Geometry: final body of the model. Coordinates: model frame, mm. Give positions to 0.01 mm unless a question says otherwise; leave off trailing zeros. Write each loop counter-clockwise with the first axis right and the second up, starting at its lowest first coordinate (ties: lowest second). Pieces come first, ordered by that corner, then holes. Notation, with made-up numbers: (-28.75, -36) - (-1.75, -36) arc R13 cw to (-1.75, -14) - close; hole circle Ø1 at (28, 46). An arc over 180 degrees is marked (long way). Return JSON: item names as keys, results as strings.
from build123d import *

# Parameters (mm, degrees)
BOSS_EXTRUDE1_DEPTH            = 9.525
CUT_EXTRUDE1_REACH             = 11.525
SKETCH2_R                      = 2.54
SKETCH2_W                      = 6.35
SKETCH2_H                      = 30
CUT_EXTRUDE2_REACH             = 230.6
SKETCH3_R                      = 2.2479
F_7_0_201_DIAMETER_HOLE1_D     = 5.1054
F_7_0_201_DIAMETER_HOLE1_DEPTH = 3.175
F_7_0_201_DIAMETER_HOLE1_TIP   = 1.533816902
SKETCH7_R                      = 6.35
CUT_EXTRUDE3_DEPTH             = 10.525


with BuildPart() as part:
    # Sketch1 → Boss-Extrude1 (new body)
    with BuildSketch(Plane(origin=(0, 0, 0), x_dir=(1, 0, 0), z_dir=(0, 1, 0))):
        with BuildLine():
            Line((6.35, 0), (101.6, 0))
            ThreePointArc((101.6, 0), (155.481536726, -22.318463274), (177.8, -76.2))
            Line((177.8, -76.2), (177.8, -228.6))
            ThreePointArc((177.8, -228.6), (203.2, -254), (228.6, -228.6))
            Line((228.6, -228.6), (228.6, 241.3))
            ThreePointArc((228.6, 241.3), (224.880256121, 250.280256121), (215.9, 254))
            Line((215.9, 254), (6.35, 254))
            ThreePointArc((6.35, 254), (1.859871939, 252.140128061), (0, 247.65))
            Line((0, 247.65), (0, 6.35))
            ThreePointArc((0, 6.35), (1.859871939, 1.859871939), (6.35, 0))
        make_face()
    extrude(amount=BOSS_EXTRUDE1_DEPTH)

    # Sketch2 → Cut-Extrude1 (cut, up to next)
    with BuildSketch(Plane(origin=(0, 9.525, 0), x_dir=(1, 0, 0), z_dir=(0, 1, 0)), mode=Mode.PRIVATE) as cut_extrude1_sk1:
        with Locations((28.34999918, 213.6)):
            Circle(SKETCH2_R)
    cut_extrude1_tool1 = extrude(cut_extrude1_sk1.sketch, amount=-CUT_EXTRUDE1_REACH, mode=Mode.PRIVATE) & part.part
    add(cut_extrude1_tool1.solids().sort_by_distance((28.349999, 9.525, -213.6))[0], mode=Mode.SUBTRACT)
    # Sketch2 → Cut-Extrude1 (cut, up to next)
    with BuildSketch(Plane(origin=(0, 9.525, 0), x_dir=(1, 0, 0), z_dir=(0, 1, 0)), mode=Mode.PRIVATE) as cut_extrude1_sk2:
        with Locations((19.3499994, 222.59999978)):
            Circle(SKETCH2_R)
    cut_extrude1_tool2 = extrude(cut_extrude1_sk2.sketch, amount=-CUT_EXTRUDE1_REACH, mode=Mode.PRIVATE) & part.part
    add(cut_extrude1_tool2.solids().sort_by_distance((19.349999, 9.525, -222.6))[0], mode=Mode.SUBTRACT)
    # Sketch2 → Cut-Extrude1 (cut, up to next)
    with BuildSketch(Plane(origin=(0, 9.525, 0), x_dir=(1, 0, 0), z_dir=(0, 1, 0)), mode=Mode.PRIVATE) as cut_extrude1_sk3:
        with Locations((19.3499994, 204.60000022)):
            Circle(SKETCH2_R)
    cut_extrude1_tool3 = extrude(cut_extrude1_sk3.sketch, amount=-CUT_EXTRUDE1_REACH, mode=Mode.PRIVATE) & part.part
    add(cut_extrude1_tool3.solids().sort_by_distance((19.349999, 9.525, -204.6))[0], mode=Mode.SUBTRACT)
    # Sketch2 → Cut-Extrude1 (cut, up to next)
    with BuildSketch(Plane(origin=(0, 9.525, 0), x_dir=(1, 0, 0), z_dir=(0, 1, 0)), mode=Mode.PRIVATE) as cut_extrude1_sk4:
        with Locations((28.34999918, 92.95)):
            Circle(SKETCH2_R)
    cut_extrude1_tool4 = extrude(cut_extrude1_sk4.sketch, amount=-CUT_EXTRUDE1_REACH, mode=Mode.PRIVATE) & part.part
    add(cut_extrude1_tool4.solids().sort_by_distance((28.349999, 9.525, -92.95))[0], mode=Mode.SUBTRACT)
    # Sketch2 → Cut-Extrude1 (cut, up to next)
    with BuildSketch(Plane(origin=(0, 9.525, 0), x_dir=(1, 0, 0), z_dir=(0, 1, 0)), mode=Mode.PRIVATE) as cut_extrude1_sk5:
        with Locations((19.3499994, 101.94999978)):
            Circle(SKETCH2_R)
    cut_extrude1_tool5 = extrude(cut_extrude1_sk5.sketch, amount=-CUT_EXTRUDE1_REACH, mode=Mode.PRIVATE) & part.part
    add(cut_extrude1_tool5.solids().sort_by_distance((19.349999, 9.525, -101.95))[0], mode=Mode.SUBTRACT)
    # Sketch2 → Cut-Extrude1 (cut, up to next)
    with BuildSketch(Plane(origin=(0, 9.525, 0), x_dir=(1, 0, 0), z_dir=(0, 1, 0)), mode=Mode.PRIVATE) as cut_extrude1_sk6:
        with Locations((19.3499994, 83.95000022)):
            Circle(SKETCH2_R)
    cut_extrude1_tool6 = extrude(cut_extrude1_sk6.sketch, amount=-CUT_EXTRUDE1_REACH, mode=Mode.PRIVATE) & part.part
    add(cut_extrude1_tool6.solids().sort_by_distance((19.349999, 9.525, -83.95))[0], mode=Mode.SUBTRACT)
    # Sketch2 → Cut-Extrude1 (cut, up to next)
    with BuildSketch(Plane(origin=(0, 9.525, 0), x_dir=(1, 0, 0), z_dir=(0, 1, 0)), mode=Mode.PRIVATE) as cut_extrude1_sk7:
        with Locations((3.175, 213.6)):
            Rectangle(SKETCH2_W, SKETCH2_H)
    cut_extrude1_tool7 = extrude(cut_extrude1_sk7.sketch, amount=-CUT_EXTRUDE1_REACH, mode=Mode.PRIVATE) & part.part
    add(cut_extrude1_tool7.solids().sort_by_distance((3.175, 9.525, -213.6))[0], mode=Mode.SUBTRACT)
    # Sketch2 → Cut-Extrude1 (cut, up to next)
    with BuildSketch(Plane(origin=(0, 9.525, 0), x_dir=(1, 0, 0), z_dir=(0, 1, 0)), mode=Mode.PRIVATE) as cut_extrude1_sk8:
        with Locations((3.175, 92.95)):
            Rectangle(SKETCH2_W, SKETCH2_H)
    cut_extrude1_tool8 = extrude(cut_extrude1_sk8.sketch, amount=-CUT_EXTRUDE1_REACH, mode=Mode.PRIVATE) & part.part
    add(cut_extrude1_tool8.solids().sort_by_distance((3.175, 9.525, -92.95))[0], mode=Mode.SUBTRACT)

    # Sketch3 → Cut-Extrude2 (cut, up to next)
    with BuildSketch(Plane(origin=(228.6, 0, 0), x_dir=(0, 0, -1), z_dir=(1, 0, 0)), mode=Mode.PRIVATE) as cut_extrude2_sk1:
        with Locations((-177.8, 4.7625)):
            Circle(SKETCH3_R)
    cut_extrude2_tool1 = extrude(cut_extrude2_sk1.sketch, amount=-CUT_EXTRUDE2_REACH, mode=Mode.PRIVATE) & part.part
    add(cut_extrude2_tool1.solids().sort_by_distance((228.6, 4.7625, 177.8))[0], mode=Mode.SUBTRACT)

    # #7 (0.201) Diameter Hole1
    with Locations(Plane(origin=(0, 0, 0), x_dir=(-1, 0, 0), z_dir=(0, -1, 0))):
        with Locations((-165.1, 143.75), (-165.1, 162.8)):
            Hole(F_7_0_201_DIAMETER_HOLE1_D / 2, depth=F_7_0_201_DIAMETER_HOLE1_DEPTH)
            with Locations((0, 0, -(F_7_0_201_DIAMETER_HOLE1_DEPTH + F_7_0_201_DIAMETER_HOLE1_TIP / 2))):  # 118° drill point
                Cone(0, F_7_0_201_DIAMETER_HOLE1_D / 2, F_7_0_201_DIAMETER_HOLE1_TIP, mode=Mode.SUBTRACT)

    # Sketch7 → Cut-Extrude3 (cut, through all)
    with BuildSketch(Plane(origin=(0, 9.525, 0), x_dir=(1, 0, 0), z_dir=(0, 1, 0))):
        with Locations((215.9, 153.275)):
            Circle(SKETCH7_R)
    extrude(amount=-CUT_EXTRUDE3_DEPTH, mode=Mode.SUBTRACT)


solid = part.part
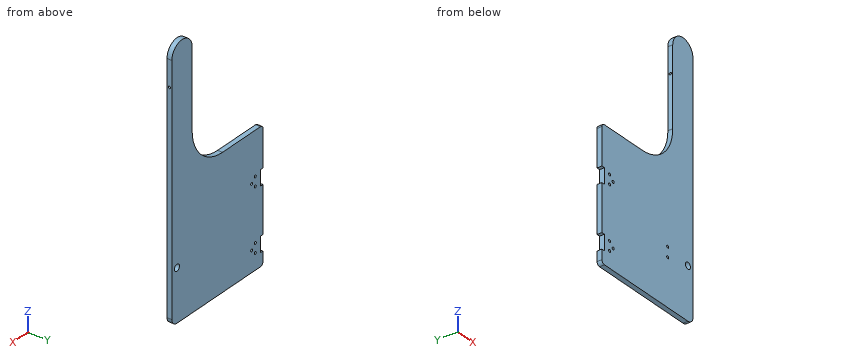
Q1. Pin query (flat end, axial travel): P1, Ø4, axis at y = 4.76, z = 177.8, coming from the +X side; P2, Ø3, axis at y = 5.5, z = -99.5, coming from the -X side; P3, Ø8, axis at x = 19.35, z = -222.6, coming from the +Y side (3 decimals); P4, Ø3, axis at x = 3, y = 5, coming from the +Z side. Return the tip coordinate at first contact, or that it passes through.
Answer key:
{"P1": "passes through", "P2": "stops at x = 6.35", "P3": "stops at y = 9.525", "P4": "stops at z = -0.28"}
Q2. Section query B-B, the plane x = 54.5. Return the cut outline in (y, z) (3 decimals), plus the area to 3 significant figures.
Answer key:
{"outline": "(0, -254) - (9.525, -254) - (9.525, 0) - (0, 0) - close", "area": "2,420 mm^2"}
Q3. Material intervals for probe 1 along Z at (x, y) = (19.35, 5.25); probe 2 along Z at (x, y) = (28.35, 6); probe 3 along X at (y, z) = (6, -92.95), sorted ascending. Write a range as [from, to].
Answer key:
{"probe 1": "z = [-254, -225.14], [-220.06, -207.14], [-202.06, -104.49], [-99.41, -86.49], [-81.41, 0]", "probe 2": "z = [-254, -216.14], [-211.06, -95.49], [-90.41, 0]", "probe 3": "x = [6.35, 25.81], [30.89, 228.6]"}
Q4. Section query A-A, the plane z = 153.5. Return the cut outline in (x, y) (3 decimals).
Answer key:
{"outline": "(177.8, 0) - (228.6, 0) - (228.6, 9.525) - (177.8, 9.525) - close"}
